```python
from build123d import *

# Parameters (mm, degrees)
SKETCH1_R                                           = 53.975
BOSS_EXTRUDE1_DEPTH                                 = 6.35
CSK_FOR_1_4_FLAT_HEAD_MACHINE_SCREW_100_D           = 6.7564
CSK_FOR_1_4_FLAT_HEAD_MACHINE_SCREW_100_CSINK_D     = 12.8778
CSK_FOR_1_4_FLAT_HEAD_MACHINE_SCREW_100_CSINK_ANGLE = 100
SKETCH4_R                                           = 53.975
SKETCH4_R_2                                         = 50.8
BOSS_EXTRUDE2_DEPTH                                 = 127


with BuildPart() as part:
    # Sketch1 → Boss-Extrude1 (new body)
    with BuildSketch(Plane.XY):
        Circle(SKETCH1_R)
    extrude(amount=BOSS_EXTRUDE1_DEPTH)

    # CSK for 1/4 Flat Head Machine Screw (100)1 (through all)
    with Locations(Plane.XY.offset(6.35)):
        with Locations((0, 0)):
            CounterSinkHole(CSK_FOR_1_4_FLAT_HEAD_MACHINE_SCREW_100_D / 2, CSK_FOR_1_4_FLAT_HEAD_MACHINE_SCREW_100_CSINK_D / 2, counter_sink_angle=CSK_FOR_1_4_FLAT_HEAD_MACHINE_SCREW_100_CSINK_ANGLE)

    # Sketch4 → Boss-Extrude2 (add)
    with BuildSketch(Plane.XY.offset(6.35)):
        Circle(SKETCH4_R)
        Circle(SKETCH4_R_2, mode=Mode.SUBTRACT)
    extrude(amount=BOSS_EXTRUDE2_DEPTH)


solid = part.part
```
Input: part model. Units: mm. Frame: model coordinates. A direction names the side the tool comes from. Give positions to 0.01 mm unless a question says otherwise; leave off trailing zeros. Order: outer loops, then holes, each group sorted by start corner. A loop starts at its lowest first (then second) coordinate and runs counter-clockwise, first axis right, second up.
1. Section C-C on y = -37. Return the cut outline in (x, z), and give its area (3 significant figures).
Derived:
outline: (-39.3, 0) - (39.3, 0) - (39.3, 133.35) - (34.81, 133.35) - (34.81, 6.35) - (-34.81, 6.35) - (-34.81, 133.35) - (-39.3, 133.35) - close
area: 1,640 mm2
2. Pin query (flat end, axial travel): pin 1 (5 mm diameter, centred on y = -34.5, z = 14, fed in from -X); pin 2 (12 mm diameter, centred on x = 36.5, z = 80.5, fed in from +Y); pin 3 (4 mm diameter, centred on x = -36.5, z = 46.5, fed in from +Y); pin 4 (4 mm diameter, centred on x = -17.5, y = -2.5, fed in from -Z). Return the tip coordinate at first contact, or that it passes through.
Derived:
pin 1: stops at x = -43.47
pin 2: stops at y = 44.53
pin 3: stops at y = 41.51
pin 4: stops at z = 0
3. Mould query, pull axis X, two halves, no side actions, for faces 1 (the flat face through (40, -32, 133.35)), 2 (the cylindrical face through (-11.012, -49.592, 68.961)), 3 (the cylindrical face through (-39.78, 36.48, 65.74)). Classes: released by +X, released by -X, zero draft, split by the parting line, or undercut.
Derived:
face 1: zero draft
face 2: undercut
face 3: split by the parting line
4. Material intervals for L1, parallel to Y at x = 0, z = 66 (3 decimals); L2, parallel to X at y = 0.5, z = 24.5; L3, parallel to Z at x = 23, y = -4.5, sorted ascending.
Derived:
L1: y = -53.975 to -50.8, 50.8 to 53.975
L2: x = -53.97 to -50.8, 50.8 to 53.97
L3: z = 0 to 6.35
5. Reachability of faces 4 (the flat face through (11, 1, 0)), 5 (the flat face through (11, 1, 6.35)) from +Z, -Z, +X, -X, +Y, -Y: full face, straight path, thin tool, end or side. Return the list, or none.
Derived:
face 4: -Z, +X, -X, +Y, -Y
face 5: +Z
6. Section A-A on x = 0. Return the cut outline in (y, z) (3 decimals), and give its area (3 significant figures).
Derived:
outline: (-53.975, 0) - (-3.378, 0) - (-3.378, 3.782) - (-6.439, 6.35) - (-50.8, 6.35) - (-50.8, 133.35) - (-53.975, 133.35) - close; (3.378, 0) - (53.975, 0) - (53.975, 133.35) - (50.8, 133.35) - (50.8, 6.35) - (6.439, 6.35) - (3.378, 3.782) - close
area: 1,440 mm2
7. Section D-D on z = 85. Return the cut outline in (x, y) (3 decimals).
Derived:
outline: circle Ø107.95 at (0, 0); hole circle Ø101.6 at (0, 0)
